from build123d import *

# Parameters (mm, degrees)
SPUR_START             = -32.726855157
SPUR_GEAR_GB_OUTLINE_R = 22.5
SPUR_GEAR_GB_DEPTH     = 75
SKETCH_2_R             = 56.152658256
CUT_EXTRUDE_1_DEPTH    = 45
EXTRUDE_1_DEPTH        = 30
EXTRUDE_START          = -30
SKETCH_5_R             = 22.5
EXTRUDE_2_DEPTH        = 30
SCALE_1_SCALE          = 0.2
CUT_EXTRUDE_3_DEPTH    = 10
EXTRUDE_3_DEPTH        = 5
SKETCH_8_R             = 1.65
CUT_EXTRUDE_4_DEPTH    = 10
SKETCH_9_W             = 18.454746183
SKETCH_9_H             = 13.449677925
CUT_EXTRUDE_5_DEPTH    = 2.5
SKETCH_10_R            = 1.446114005
SKETCH_10_R_2          = 1.567494057
SKETCH_10_R_3          = 1.749983797
SKETCH_10_R_4          = 1.35600832
CUT_EXTRUDE_6_DEPTH    = 80.014451116


# Read off the part's stored shape, not the designer's step: spur gear_gb
with BuildPart() as part:
    # spur gear_gb outline → spur gear_gb (new body)
    with BuildSketch(Plane.YZ.offset(SPUR_START)):
        with BuildLine():
            ThreePointArc((32.862431273, 33.858374177), (32.001554259, 34.671025411), (31.120587981, 35.461853886))
            ThreePointArc((31.120587981, 35.461853886), (26.170323532, 33.302671085), (22.140322459, 29.707357493))
            ThreePointArc((22.140322459, 29.707357493), (20.304903422, 30.987038971), (18.395725829, 32.153824573))
            ThreePointArc((18.395725829, 32.153824573), (20.069385125, 37.288613083), (20.058208562, 42.689267077))
            ThreePointArc((20.058208562, 42.689267077), (18.980108815, 43.178360316), (17.890094133, 43.64029024))
            ThreePointArc((17.890094133, 43.64029024), (13.909134176, 39.99074968), (11.264886092, 35.281700885))
            ThreePointArc((11.264886092, 35.281700885), (9.113403224, 35.896086104), (6.928815473, 36.379743093))
            ThreePointArc((6.928815473, 36.379743093), (6.844528189, 41.779750883), (5.080367717, 46.884153523))
            ThreePointArc((5.080367717, 46.884153523), (3.901874073, 46.996687926), (2.720930993, 47.079662024))
            ThreePointArc((2.720930993, 47.079662024), (0.14067431, 42.335248053), (-0.831275476, 37.022762562))
            ThreePointArc((-0.831275476, 37.022762562), (-3.065675621, 36.90527335), (-5.28893955, 36.653389986))
            ThreePointArc((-5.28893955, 36.653389986), (-7.12203958, 41.733442422), (-10.448009799, 45.988452479))
            ThreePointArc((-10.448009799, 45.988452479), (-11.599189267, 45.712233197), (-12.74308724, 45.407259939))
            ThreePointArc((-12.74308724, 45.407259939), (-13.643029801, 40.082103428), (-12.837355447, 34.741871474))
            ThreePointArc((-12.837355447, 34.741871474), (-14.912540945, 33.90523961), (-16.933555907, 32.945111364))
            ThreePointArc((-16.933555907, 32.945111364), (-20.316823851, 37.154705941), (-24.844183336, 40.099227051))
            ThreePointArc((-24.844183336, 40.099227051), (-25.843300471, 39.464186729), (-26.826194241, 38.804314699))
            ThreePointArc((-26.826194241, 38.804314699), (-25.948299939, 33.475478984), (-23.452308764, 28.686197563))
            ThreePointArc((-23.452308764, 28.686197563), (-25.143401065, 27.221085091), (-26.74315873, 25.656756756))
            ThreePointArc((-26.74315873, 25.656756756), (-31.309965009, 28.539718582), (-36.548104111, 29.854666195))
            ThreePointArc((-36.548104111, 29.854666195), (-37.286889069, 28.929621306), (-38.002266845, 27.986357877))
            ThreePointArc((-38.002266845, 27.986357877), (-35.44166915, 23.231304993), (-31.525840525, 19.51196706))
            ThreePointArc((-31.525840525, 19.51196706), (-32.64958354, 17.577141651), (-33.654725342, 15.578132475))
            ThreePointArc((-33.654725342, 15.578132475), (-38.910185635, 16.822047902), (-44.291470704, 16.364927041))
            ThreePointArc((-44.291470704, 16.364927041), (-44.68986467, 15.250120552), (-45.060204171, 14.125682952))
            ThreePointArc((-45.060204171, 14.125682952), (-41.094383574, 10.459696662), (-36.183058293, 8.213350193))
            ThreePointArc((-36.183058293, 8.213350193), (-36.617677028, 6.018480201), (-36.919280256, 3.801413847))
            ThreePointArc((-36.919280256, 3.801413847), (-42.293883893, 3.271485337), (-47.235169193, 1.091832139))
            ThreePointArc((-47.235169193, 1.091832139), (-47.25, -0.091929368), (-47.235169193, -1.275690876))
            ThreePointArc((-47.235169193, -1.275690876), (-42.293883893, -3.455344074), (-36.919280256, -3.985272584))
            ThreePointArc((-36.919280256, -3.985272584), (-36.617677028, -6.202338938), (-36.183058293, -8.39720893))
            ThreePointArc((-36.183058293, -8.39720893), (-41.094383574, -10.643555399), (-45.060204171, -14.309541689))
            ThreePointArc((-45.060204171, -14.309541689), (-44.68986467, -15.433979288), (-44.291470704, -16.548785777))
            ThreePointArc((-44.291470704, -16.548785777), (-38.910185635, -17.005906639), (-33.654725342, -15.761991212))
            ThreePointArc((-33.654725342, -15.761991212), (-32.64958354, -17.761000388), (-31.525840525, -19.695825796))
            ThreePointArc((-31.525840525, -19.695825796), (-35.44166915, -23.41516373), (-38.002266845, -28.170216613))
            ThreePointArc((-38.002266845, -28.170216613), (-37.286889069, -29.113480043), (-36.548104111, -30.038524932))
            ThreePointArc((-36.548104111, -30.038524932), (-31.309965009, -28.723577319), (-26.74315873, -25.840615493))
            ThreePointArc((-26.74315873, -25.840615493), (-25.143401065, -27.404943828), (-23.452308764, -28.870056299))
            ThreePointArc((-23.452308764, -28.870056299), (-25.948299939, -33.65933772), (-26.826194241, -38.988173435))
            ThreePointArc((-26.826194241, -38.988173435), (-25.843300471, -39.648045466), (-24.844183336, -40.283085788))
            ThreePointArc((-24.844183336, -40.283085788), (-20.316823851, -37.338564677), (-16.933555907, -33.128970101))
            ThreePointArc((-16.933555907, -33.128970101), (-14.912540945, -34.089098347), (-12.837355447, -34.925730211))
            ThreePointArc((-12.837355447, -34.925730211), (-13.643029801, -40.265962164), (-12.74308724, -45.591118675))
            ThreePointArc((-12.74308724, -45.591118675), (-11.599189267, -45.896091934), (-10.448009799, -46.172311216))
            ThreePointArc((-10.448009799, -46.172311216), (-7.12203958, -41.917301159), (-5.28893955, -36.837248723))
            ThreePointArc((-5.28893955, -36.837248723), (-3.065675621, -37.089132087), (-0.831275476, -37.206621299))
            ThreePointArc((-0.831275476, -37.206621299), (0.14067431, -42.51910679), (2.720930993, -47.263520761))
            ThreePointArc((2.720930993, -47.263520761), (3.901874073, -47.180546663), (5.080367717, -47.06801226))
            ThreePointArc((5.080367717, -47.06801226), (6.844528189, -41.96360962), (6.928815473, -36.56360183))
            ThreePointArc((6.928815473, -36.56360183), (9.113403224, -36.079944841), (11.264886092, -35.465559622))
            ThreePointArc((11.264886092, -35.465559622), (13.909134176, -40.174608417), (17.890094133, -43.824148977))
            ThreePointArc((17.890094133, -43.824148977), (18.980108815, -43.362219053), (20.058208562, -42.873125814))
            ThreePointArc((20.058208562, -42.873125814), (20.069385125, -37.47247182), (18.395725829, -32.33768331))
            ThreePointArc((18.395725829, -32.33768331), (20.304903422, -31.170897707), (22.140322459, -29.891216229))
            ThreePointArc((22.140322459, -29.891216229), (26.170323532, -33.486529822), (31.120587981, -35.645712623))
            ThreePointArc((31.120587981, -35.645712623), (32.001554259, -34.854884148), (32.862431273, -34.042232914))
            ThreePointArc((32.862431273, -34.042232914), (31.119412774, -28.930572226), (27.869173851, -24.617437006))
            ThreePointArc((27.869173851, -24.617437006), (29.296052271, -22.893962115), (30.616511345, -21.087657722))
            ThreePointArc((30.616511345, -21.087657722), (35.595552259, -23.179628097), (40.978683235, -23.614472179))
            ThreePointArc((40.978683235, -23.614472179), (41.555134745, -22.58044369), (42.105499643, -21.532297832))
            ThreePointArc((42.105499643, -21.532297832), (38.797169181, -17.2635582), (34.322564452, -14.239471396))
            ThreePointArc((34.322564452, -14.239471396), (35.112519281, -12.146072463), (35.774926162, -10.008886264))
            ThreePointArc((35.774926162, -10.008886264), (41.163450577, -10.370815972), (46.396102311, -9.034199232))
            ThreePointArc((46.396102311, -9.034199232), (46.605571586, -7.869023759), (46.785783792, -6.698966145))
            ThreePointArc((46.785783792, -6.698966145), (42.270650308, -3.735731746), (37.056572625, -2.328400087))
            ThreePointArc((37.056572625, -2.328400087), (37.124, -0.091929368), (37.056572625, 2.14454135))
            ThreePointArc((37.056572625, 2.14454135), (42.270650308, 3.551873009), (46.785783792, 6.515107408))
            ThreePointArc((46.785783792, 6.515107408), (46.605571586, 7.685165023), (46.396102311, 8.850340496))
            ThreePointArc((46.396102311, 8.850340496), (41.163450577, 10.186957235), (35.774926162, 9.825027527))
            ThreePointArc((35.774926162, 9.825027527), (35.112519281, 11.962213726), (34.322564452, 14.05561266))
            ThreePointArc((34.322564452, 14.05561266), (38.797169181, 17.079699464), (42.105499643, 21.348439095))
            ThreePointArc((42.105499643, 21.348439095), (41.555134745, 22.396584953), (40.978683235, 23.430613443))
            ThreePointArc((40.978683235, 23.430613443), (35.595552259, 22.99576936), (30.616511345, 20.903798985))
            ThreePointArc((30.616511345, 20.903798985), (29.296052271, 22.710103378), (27.869173851, 24.433578269))
            ThreePointArc((27.869173851, 24.433578269), (31.119412774, 28.746713489), (32.862431273, 33.858374177))
        make_face()
        with Locations((0, -0.091929368)):
            Circle(SPUR_GEAR_GB_OUTLINE_R, mode=Mode.SUBTRACT)
    extrude(amount=SPUR_GEAR_GB_DEPTH)

    # 草图2 → 切除-拉伸1 (cut)
    with BuildSketch(Plane.ZY.offset(32.726855157)):
        with Locations((-0.091929368, 0)):
            Circle(SKETCH_2_R)
    extrude(amount=-CUT_EXTRUDE_1_DEPTH, mode=Mode.SUBTRACT)

    # 草图4 → 凸台-拉伸1 (add)
    with BuildSketch(Plane(origin=(42.273144843, 0, 0), x_dir=(0, 0, -1), z_dir=(1, 0, 0))):
        with BuildLine():
            Line((-24.433578269, 27.869173851), (-23.430613443, 40.978683235))
            Line((-23.430613443, 40.978683235), (-14.487711984, 157.869173851))
            ThreePointArc((-14.487711984, 157.869173851), (7.042421291, 176.339040577), (25.512288016, 154.808907302))
            Line((25.512288016, 154.808907302), (24.617437006, 27.869173851))
            Line((24.617437006, 27.869173851), (-24.433578269, 27.869173851))
        make_face()
    extrude(amount=-EXTRUDE_1_DEPTH)

    # 草图5 → 凸台-拉伸2 (add)
    with BuildSketch(Plane(origin=(42.273144843, 0, 0), x_dir=(0, 0, -1), z_dir=(1, 0, 0)).offset(EXTRUDE_START)):
        with Locations((0.091929368, 0)):
            Circle(SKETCH_5_R)
    extrude(amount=EXTRUDE_2_DEPTH)


with BuildPart() as part_1:
    # 缩放比例1: scaled about (27.273144843, 52.936955481, -1.705643422)
    add(part.part.scale(SCALE_1_SCALE).moved(Location((21.818515874, 42.349564385, -1.364514738))))

    # 草图6 → 切除-拉伸3 (cut)
    with BuildSketch(Plane(origin=(30.273144843, 0, 0), x_dir=(0, 0, -1), z_dir=(1, 0, 0))):
        with BuildLine():
            ThreePointArc((1.382900611, 38.849564385), (4.342900611, 44.217290275), (-1.776224322, 43.856192956))
            ThreePointArc((-1.776224322, 43.856192956), (-1.577099389, 40.481838495), (1.382900611, 38.849564385))
        make_face()
    extrude(amount=-CUT_EXTRUDE_3_DEPTH, mode=Mode.SUBTRACT)

    # 草图7 → 凸台-拉伸3 (add, symmetric)
    with BuildSketch(Plane(origin=(27.273144843, 0, 0), x_dir=(0, 0, -1), z_dir=(1, 0, 0))):
        with BuildLine():
            Line((6.288002139, 47.923399155), (6.466972341, 73.311345845))
            ThreePointArc((6.466972341, 73.311345845), (2.772998996, 77.6173725), (-1.533027659, 73.923399155))
            Line((-1.533027659, 73.923399155), (-3.321607951, 50.545301032))
            Line((-3.321607951, 50.545301032), (-3.322451181, 50.53427937))
            Line((-3.322451181, 50.53427937), (-3.522200916, 47.923399155))
            Line((-3.522200916, 47.923399155), (6.288002139, 47.923399155))
        make_face()
    extrude(amount=EXTRUDE_3_DEPTH, both=True)

    # 草图8 → 切除-拉伸4 (cut)
    with BuildSketch(Plane(origin=(32.273144843, 0, 0), x_dir=(0, 0, -1), z_dir=(1, 0, 0))):
        with Locations((2.466972341, 73.6173725)):
            Circle(SKETCH_8_R)
    extrude(amount=-CUT_EXTRUDE_4_DEPTH, mode=Mode.SUBTRACT)

    # 草图9 → 切除-拉伸5 (cut, symmetric)
    with BuildSketch(Plane(origin=(27.273144843, 0, 0), x_dir=(0, 0, -1), z_dir=(1, 0, 0))):
        with Locations((1.880211444, 72.900415106)):
            Rectangle(SKETCH_9_W, SKETCH_9_H)
    extrude(amount=CUT_EXTRUDE_5_DEPTH, both=True, mode=Mode.SUBTRACT)

    # 草图10 → 切除-拉伸6 (cut, through all)
    with BuildSketch(Plane(origin=(32.273144843, 0, 0), x_dir=(0, 0, -1), z_dir=(1, 0, 0))):
        with Locations((0.89588905, 50.944816989)):
            Circle(SKETCH_10_R)
        with Locations((1.285013172, 55.613074907)):
            Circle(SKETCH_10_R_2)
        with Locations((1.667330314, 59.914483987)):
            Circle(SKETCH_10_R_3)
        with Locations((2.056454436, 64.582741905)):
            Circle(SKETCH_10_R_4)
    extrude(amount=-CUT_EXTRUDE_6_DEPTH, mode=Mode.SUBTRACT)


solid = part_1.part
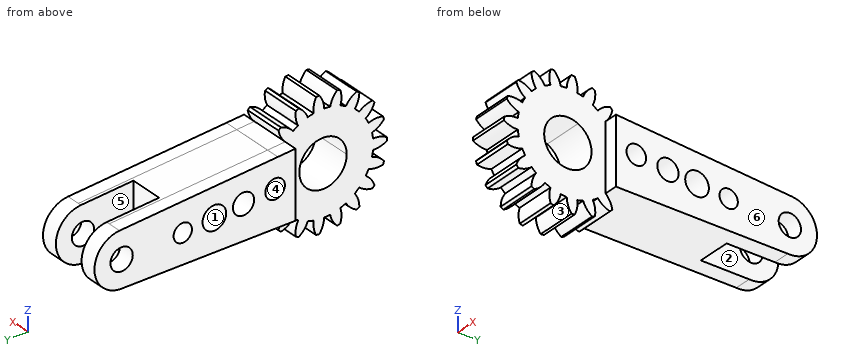
Could you check a few things on this model? Use its own coordinates, in mm. Face numbers are marked on the shaded views. A direction names the side the tool comes from. Coordinates: 2 decimals unless noted, no trailing zeros. Write each loop counter-clockwise with the first axis right and the second up, starting at its lowest first coordinate (ties: lowest second). Pieces come first, ordered by that corner, then holes. Notation, with made-up numbers: (-39.5, 19) - (-32.5, 19) arc R5 cw to (-32.5, 28) - close; hole circle Ø2 at (-37, 65.5). An arc over 180 degrees is marked (long way). Write item = value, one per line.
1) Suppose I cut it at B-B on y = 36.5. Please give me the cut outline in (x, z), plus the area to 3 significant figures.
Result set:
outline = (24.27, -6.9) - (30.27, -6.9) - (30.27, 4.13) - (24.27, 4.13) - close
area = 66.2 mm2
2) For the marked faces 5 and 6, which set-ups out of +Z, -Z, +X, -X, +Y, -Y let a thin tool reach every point of the face, with its end or its side?
Result set:
face_5 = +Z, -Z, +Y
face_6 = +Z, -Z, +X, +Y, -Y
3) Suppose I cut it at A-A on x = 28.75. State how many separate pieces and enclosed holes the cut face has, plus the area to 3 significant figures.
Result set:
separate_pieces = 1
enclosed_holes = 5
area = 298 mm2
4) Will these pins go through, and if not, where does the flat tip stop? pin 1 Ø11 at (y, z) = (42.35, -1.38) entering from +X; pin 2 Ø1 at (x, z) = (31.5, -3) entering from -Y; pin 3 Ø2.5 at (y, z) = (73.62, -2.47) entering from -X; pin 4 Ø5 at (x, y) = (28.5, 71.5) entering from +Z.
Result set:
pin_1 = 30.27
pin_2 = 47.92
pin_3 = through
pin_4 = 1.88
5) Please list where these lines run through material, in increasing order: line 1 (X direction, y = 68.5, z = -5); line 2 (Y direction, x = 31, z = -3); line 3 (Y direction, x = 27, z = -3). Write a range as [from, to].
Result set:
line_1 = [22.27, 24.77], [29.77, 32.27]
line_2 = [47.92, 58.78], [61.05, 63.61], [65.56, 72.06], [75.18, 77.59]
line_3 = [35.1, 39.25], [45.45, 58.78], [61.05, 63.61], [65.56, 66.18]
6) We'd pull the mould along Z, two halves only. Please class the marked faces 1, 2, 3 and 4: +Z half, -Z half, draft (parallel to the pull), parting line (faces both ways), or undercut.
Result set:
face_1 = undercut
face_2 = draft
face_3 = -Z half
face_4 = undercut
